Geometry check sheet. Reference: the model listing, model coordinates, mm. Face numbers are marked on the shaded views. Round coordinates to 2 decimals unless told otherwise and drop trailing zeros. Order: outer loops, then holes, each group sorted by start corner. A loop starts at its lowest first (then second) coordinate and runs counter-clockwise, first axis right, second up.
```python
from build123d import *

# Parameters (mm, degrees)
F1_DEPTH = 5
F3_DEPTH = 1
F5_DEPTH = 1


with BuildPart() as f1:
    # F0 (on Top) → F1 (new body)
    with BuildSketch(Plane.XY):
        Polygon((18.706655, 7.32937), (12.535754, 15.700748), (3.005907, 19.865124), (-7.32937, 18.706655), (-15.700748, 12.535754), (-19.865124, 3.005907), (-18.706655, -7.32937), (-12.535754, -15.700748), (-3.005907, -19.865124), (7.32937, -18.706655), (15.700748, -12.535754), (19.865124, -3.005907), align=None)
    extrude(amount=F1_DEPTH)

    # F2 (on face) → F3 (join)
    with BuildSketch(Plane(origin=(-2.161731, 19.285889, 0), x_dir=(-0.993777, -0.111391, 0), z_dir=(-0.111391, 0.993777, 0))):
        Polygon((1, 3.5), (0, 3.5), (-1, 3.5), (-1, 1.5), (0, 1.5), (1, 1.5), align=None)
    extrude(amount=F3_DEPTH)

    # F4 (on face) → F5 (join)
    with BuildSketch(Plane(origin=(2.161731, -19.285889, 0), x_dir=(0.993777, 0.111391, 0), z_dir=(0.111391, -0.993777, 0))):
        Polygon((1, 3.5), (0, 3.5), (-1, 3.5), (-1, 1.597076), (1, 1.597076), align=None)
    extrude(amount=F5_DEPTH)


solid = f1.part
```
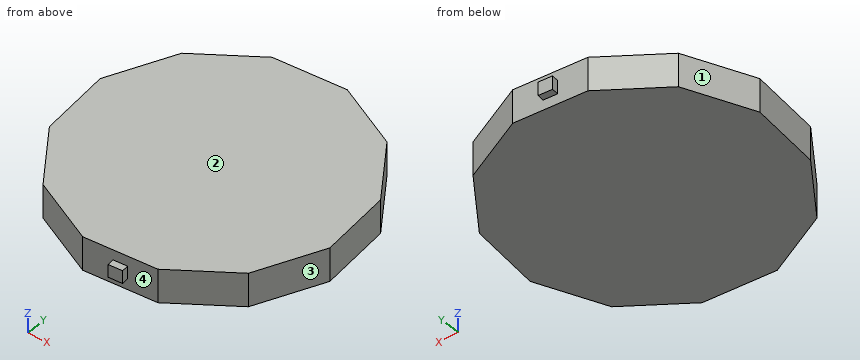
(1) Sectioned sample at C-C, the plane x = -2.5. Record the cut outline in (y, z), and give its area (3 significant figures).
Returned:
outline: (-19.81, 0) - (19.25, 0) - (19.25, 1.5) - (20.25, 1.5) - (20.25, 3.5) - (19.25, 3.5) - (19.25, 5) - (-19.81, 5) - close
area: 197 mm2
(2) Sectioned sample at D-D, the plane y = 16.5. Record the cut outline in (x, z).
Returned:
outline: (-10.32, 0) - (10.71, 0) - (10.71, 5) - (-10.32, 5) - close
(3) Sectioned sample at A-A, the plane x = 2.5. Record the cut outline in (y, z).
Returned:
outline: (-20.25, 1.6) - (-19.25, 1.6) - (-19.25, 0) - (19.81, 0) - (19.81, 5) - (-19.25, 5) - (-19.25, 3.5) - (-20.25, 3.5) - close
(4) Material ranges on line 1 (Y direction, x = 2, z = 0.6); line 2 (Y direction, x = -1, z = 1.9); line 3 (X direction, y = 18.5, z = 3.85), recorded low to high.
Returned:
line 1: y = -19.3 to 19.75
line 2: y = -19.64 to 19.42
line 3: x = -7.61 to 6.13
(5) Sectioned sample at B-B, the plane y = -2. Record the cut outline in (x, z), and give its area (3 significant figures).
Returned:
outline: (-19.3, 0) - (19.75, 0) - (19.75, 5) - (-19.3, 5) - close
area: 195 mm2
(6) Draft check along X on the marked faces 1, 2, 3 and 4. Enter one of: released by +X, released by -X, zero draft, split by the parting line, or undercut.
Returned:
face 1: released by -X
face 2: zero draft
face 3: released by +X
face 4: undercut
(7) Depth check by flat-ended pin: P1, Ø1, axis at x = -2, y = 20, coming from the +Z side; P2, Ø1, axis at x = -10.5, z = 3, coming from the -Y side; P3, Ø1.5, axis at y = -5.5, z = 1, coming from the +X side. Enter the tip coordinate at first touch or a pass-through.
Returned:
P1: stops at z = 3.5
P2: stops at y = -16.81
P3: stops at x = 19.1
